```python
from build123d import *

# Parameters (mm, degrees)
F0_R     = 6
F1_DEPTH = 3
F2_R     = 3.5
F3_DEPTH = 30


# Not quite as in the source:
# - a fillet or chamfer that OpenCascade refuses, or shapes differently, is made with other operations: its cross-section is extruded or revolved along the edge and cut away or added


with BuildPart() as f1:
    # F0 (on Top) → F1 (new body)
    with BuildSketch(Plane.XY):
        Circle(F0_R)
    extrude(amount=F1_DEPTH)

    # F2 (on face) → F3 (join)
    with BuildSketch(Plane.XY.offset(3)):
        Circle(F2_R)
    extrude(amount=F3_DEPTH)

    # F4: fillet of radius 3 on 2 edges, made by hand

    # F4_s1 → F4_t2 (revolve)
    with BuildSketch(Plane.XZ):
        with BuildLine():
            ThreePointArc((6, 3), (4.2087121525, 4.0215482184), (3.5, 5.9580398916))
            Line((3.5, 5.9580398916), (3.5, 3))
            Line((3.5, 3), (6, 3))
        make_face()
    revolve(axis=Axis((0, 0, 3), (0, 0, 1)))

    # F4_s3 → F4_t4 (revolve, cut)
    with BuildSketch(Plane.XZ):
        with BuildLine():
            ThreePointArc((3.5, 30), (2.6213203436, 32.1213203436), (0.5, 33))
            Line((0.5, 33), (3.5, 33))
            Line((3.5, 33), (3.5, 30))
        make_face()
    revolve(axis=Axis((0, 0, 33), (0, 0, 1)), mode=Mode.SUBTRACT)


solid = f1.part
```
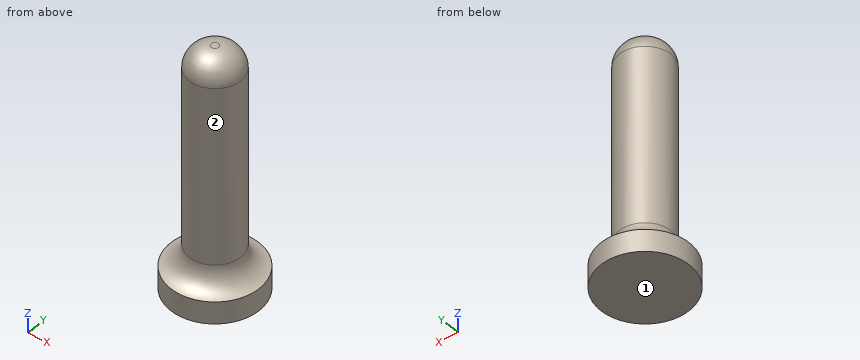
Could you check a few things on this model? Use its own coordinates, in mm. Face numbers are marked on the shaded views. A direction names the side the tool comes from. Give positions to 0.01 mm unless a question says otherwise; leave off trailing zeros. Loops run counter-clockwise (first coordinate to the right, second up) from the corner with the lowest first, then second, coordinate; pieces in that order, holes last. Notation, with made-up numbers: (-16.75, -1.75) - (6.25, -1.75) arc R11 ccw to (6.25, 18.25) - close; hole circle Ø3 at (65, 35). An arc over 180 degrees is marked (long way). Answer in a Markdown table with one row per item. Add a question column.
Q1. Which directions (+Z, -Z, +X, -X, +Y, -Y) give clear straight access to the entire face, cutting with the end or side of a thin tool? Please do the marked faces 1 and 2.
Q2. Please list where these lines run through material, in increasing order: L1, parallel to Z at x = 0.75, y = 1.5; L2, parallel to X at y = -1.5, z = 14; L3, parallel to Z at x = 4.25, y = -3.25. Write a range as from..to.
Q3. If we section it at A-A (z = 19): List the corners of the cut face in (x, y) for me, plus the area to 3 significant figures.
Q4. For pin 1 (1 mm diameter, centred on x = -1.5, z = 23.5, fed in from -Y); pin 2 (1 mm diameter, centred on x = 3, y = 0, fed in from +Z); pin 3 (6 mm diameter, centred on y = 3.5, z = 14.5, fed in from -X), each with a flat end and sliding along its axis, tell me the tip position at first contact or that it passes through.
The answers:
| question | item | result |
|---|---|---|
| 1 | face 1 | -Z, +X, -X, +Y, -Y |
| 1 | face 2 | +Z |
| 2 | L1 | z = 0..32.76 |
| 2 | L2 | x = -3.16..3.16 |
| 2 | L3 | z = 0..3.19 |
| 3 | outline | circle Ø7 at (0, 0) |
| 3 | area | 38.5 mm^2 |
| 4 | pin 1 | stops at y = -3.35 |
| 4 | pin 2 | stops at z = 32.24 |
| 4 | pin 3 | stops at x = -3.46 |
